Source: CAD feature listing. Evaluate the final solid. Frame: model axes, mm. A direction names the side the tool comes from. Give positions to 0.01 mm unless a question says otherwise; leave off trailing zeros. Loops run counter-clockwise (first coordinate to the right, second up) from the corner with the lowest first, then second, coordinate; pieces in that order, holes last.
```python
from build123d import *

# Parameters (mm, degrees)
MORS_AMOVIBLE_DEPTH     = 40
ESQUISSE2_R             = 2.4
TROU_FIXATION_DEPTH     = 6
CONG_1_R                = 5
ENL_V_START             = -40
ESQUISSE3_W             = 60
ESQUISSE3_H             = 1
ENL_V_MAT_EXTRU_1_DEPTH = 40


with BuildPart() as part:
    # Esquisse1 → mors_amovible (new body)
    with BuildSketch(Plane.XY):
        with BuildLine():
            Line((60, 0), (60, 5))
            Line((60, 5), (45, 5))
            ThreePointArc((45, 5), (30, 20), (15, 5))
            Line((15, 5), (0, 5))
            Line((0, 5), (0, 0))
            Line((0, 0), (19, 0))
            ThreePointArc((19, 0), (30, 11), (41, 0))
            Line((41, 0), (60, 0))
        make_face()
    extrude(amount=MORS_AMOVIBLE_DEPTH)

    # Esquisse2 → trou_fixation (cut, through all)
    with BuildSketch(Plane(origin=(0, 5, 0), x_dir=(1, 0, 0), z_dir=(0, 1, 0))):
        with Locations((5, -10)):
            Circle(ESQUISSE2_R)
        with Locations((55, -10)):
            Circle(ESQUISSE2_R)
        with Locations((55, -30)):
            Circle(ESQUISSE2_R)
        with Locations((5, -30)):
            Circle(ESQUISSE2_R)
    extrude(amount=-TROU_FIXATION_DEPTH, mode=Mode.SUBTRACT)

    # Congé1
    cong_1_edges = [part.edges().sort_by_distance(p)[0] for p in [
        (15, 5, 20),
        (45, 5, 20),
    ]]
    fillet(cong_1_edges, radius=CONG_1_R)

    # Esquisse3 → Enlèv. mat.-Extru.1 (cut)
    with BuildSketch(Plane(origin=(0, 0, 0), x_dir=(-1, 0, 0), z_dir=(0, 0, -1)).offset(ENL_V_START)):
        with Locations((-30, 0.5)):
            Rectangle(ESQUISSE3_W, ESQUISSE3_H)
    extrude(amount=ENL_V_MAT_EXTRU_1_DEPTH, mode=Mode.SUBTRACT)


solid = part.part
```
(1) Section D-D, the plane x = 42. Return the cut outline in (y, z), then the cut area to 3 significant figures.
A:
outline: (1, 0) - (14, 0) - (14, 40) - (1, 40) - close
area: 520 mm2
(2) Section B-B, the plane z = 30. Return the cut outline in (x, y), then the cut area to 3 significant figures.
A:
outline: (0, 1) - (2.6, 1) - (2.6, 5) - (0, 5) - close; (7.4, 1) - (19.05, 1) arc R11 cw to (40.95, 1) - (52.6, 1) - (52.6, 5) - (49.36, 5) arc R5 cw to (44.52, 8.75) arc R15 ccw to (15.48, 8.75) arc R5 cw to (10.64, 5) - (7.4, 5) - close; (57.4, 1) - (60, 1) - (60, 5) - (57.4, 5) - close
area: 394 mm2
(3) First-contact query: pin 1 (5.5 mm diameter, centred on x = 3, z = 22.5, fed in from +Y); pin 2 (4 mm diameter, centred on x = 25, z = 9, fed in from +Y); pin 3 (6 mm diameter, centred on y = 16, z = 15.5, fed in from +X). Flat tips, straight axial feed; report the tip coordinate or a pass-through.
A:
pin 1: stops at y = 5
pin 2: stops at y = 19.7
pin 3: stops at x = 42.69
(4) Mould query, pull axis X, two halves, no side actions, for faces 1 (the cylindrical face through (56.11, 3.03, 32.13)), 2 (the flat face through (30, 13, 40)), 3 (the flat face through (0, 3, 20)). Classes: pulls with the +X half, pulls with the -X half, needs draft (parallel to the pull), parting line crosses it, or undercut.
A:
face 1: undercut
face 2: needs draft
face 3: pulls with the -X half
(5) Reachability of faces 4 (the flat face through (55, 5, 20)), 5 (the flat face through (30, 13, 0)), 6 (the flat face through (5, 5, 20)) from +Z, -Z, +X, -X, +Y, -Y: full face, straight path, thin tool, end or side. Return the list, or none.
A:
face 4: +Z, -Z, +X, +Y
face 5: -Z, +X, -X, +Y, -Y
face 6: +Z, -Z, -X, +Y
(6) Section C-C, the plane z = 18. Return the cut outline in (x, y), then the cut area to 3 significant figures.
A:
outline: (0, 1) - (19.05, 1) arc R11 cw to (40.95, 1) - (60, 1) - (60, 5) - (49.36, 5) arc R5 cw to (44.52, 8.75) arc R15 ccw to (15.48, 8.75) arc R5 cw to (10.64, 5) - (0, 5) - close
area: 432 mm2
(7) Section A-A, the plane x = 55. Return the cut outline in (y, z).
A:
outline: (1, 0) - (5, 0) - (5, 7.6) - (1, 7.6) - close; (1, 12.4) - (5, 12.4) - (5, 27.6) - (1, 27.6) - close; (1, 32.4) - (5, 32.4) - (5, 40) - (1, 40) - close
(8) Ray query, line 1 along Z through (x, y) = (5, 2.6); line 2 along X through (y, z) = (2.4, 30); line 3 along X through (y, z) = (2.1, 10). Return the intervals inside material, ascending.
A:
line 1: z = 0 to 7.6, 12.4 to 27.6, 32.4 to 40
line 2: x = 0 to 2.6, 7.4 to 19.27, 40.73 to 52.6, 57.4 to 60
line 3: x = 0 to 2.6, 7.4 to 19.2, 40.8 to 52.6, 57.4 to 60
